Input: part model. Units: mm. Frame: model coordinates. Face numbers are marked on the shaded views. A direction names the side the tool comes from. Give positions to 0.01 mm unless a question says otherwise; leave off trailing zeros. Loops run counter-clockwise (first coordinate to the right, second up) from the corner with the lowest first, then second, coordinate; pieces in that order, holes last.
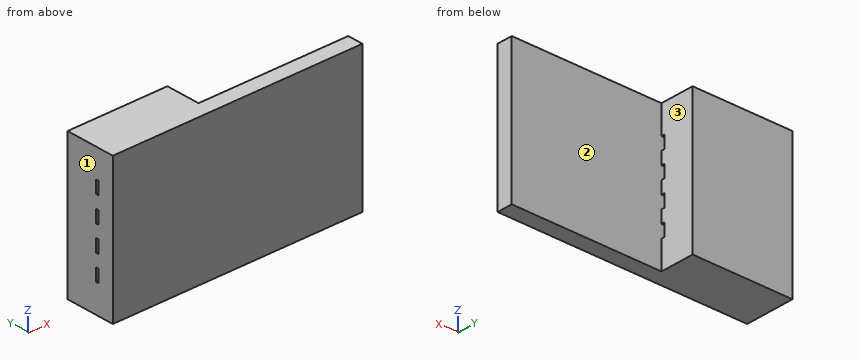
from build123d import *

# Parameters (mm, degrees)
INSULATOR_BODY_SKETCH_W    = 11.5
INSULATOR_BODY_SKETCH_H    = 4
INSULATOR_BODY_DEPTH       = 20
INSULATOR_TONGUE_SKETCH_W  = 12
INSULATOR_TONGUE_SKETCH_H  = 11.5
INSULATOR_TONGUE_DEPTH     = 2.75
CONTACT_SLOT_SKETCH_W      = 1
CONTACT_SLOT_SKETCH_H      = 0.25
CONTACT_SLOT_DEPTH         = 9
CONTACT_SLOT_PATTERN_COUNT = 4
CONTACT_SLOT_PATTERN_PITCH = 2


with BuildPart() as part:
    # Insulator_body_sketch → Insulator_body (new body)
    with BuildSketch(Plane(origin=(0, 0, 0), x_dir=(0, 0, -1), z_dir=(1, 0, 0))):
        Rectangle(INSULATOR_BODY_SKETCH_W, INSULATOR_BODY_SKETCH_H)
    extrude(amount=-INSULATOR_BODY_DEPTH)

    # Insulator_tongue_sketch → Insulator_tongue (cut)
    with BuildSketch(Plane(origin=(0, 2, 0), x_dir=(1, 0, 0), z_dir=(0, 1, 0))):
        with Locations((-6, 0)):
            Rectangle(INSULATOR_TONGUE_SKETCH_W, INSULATOR_TONGUE_SKETCH_H)
    extrude(amount=-INSULATOR_TONGUE_DEPTH, mode=Mode.SUBTRACT)

    # Contact_slot_sketch → Contact_slot (cut, through all)
    with BuildSketch(Plane(origin=(-12, 0, 0), x_dir=(0, 0, -1), z_dir=(1, 0, 0))):
        with Locations((-3, -0.625)):
            Rectangle(CONTACT_SLOT_SKETCH_W, CONTACT_SLOT_SKETCH_H)
    contact_slot = extrude(amount=-CONTACT_SLOT_DEPTH, mode=Mode.SUBTRACT)

    # Contact_slot_pattern: Contact_slot ×4
    with Locations(*[(0, 0, -i * CONTACT_SLOT_PATTERN_PITCH) for i in range(1, CONTACT_SLOT_PATTERN_COUNT)]):
        add(contact_slot, mode=Mode.SUBTRACT)


solid = part.part
(1) Cut plane C-C (y = 0.3). Return the cut outline in (x, z).
Values follow:
outline: (-20, -5.75) - (-12, -5.75) - (-12, 5.75) - (-20, 5.75) - close
(2) Cut plane D-D (x = -3.25). Return the cut outline in (y, z), and give its area (3 significant figures).
Values follow:
outline: (-2, -5.75) - (-0.75, -5.75) - (-0.75, 5.75) - (-2, 5.75) - close
area: 14.4 mm2
(3) Cut plane A-A (z = -1.25). Return the cut outline in (x, y).
Values follow:
outline: (-20, -2) - (0, -2) - (0, -0.75) - (-20, -0.75) - close; (-20, -0.5) - (-12, -0.5) - (-12, 2) - (-20, 2) - close
(4) Ray query, probe 1 along Z at (x, y) = (-14, -0.6); probe 2 along Y at (x, z) = (-17.5, 3); probe 3 along Y at (x, z) = (-2.5, 4.5). Return the intervals inside material, ascending.
Values follow:
probe 1: z = -5.75 to -3.5, -2.5 to -1.5, -0.5 to 0.5, 1.5 to 2.5, 3.5 to 5.75
probe 2: y = -2 to -0.75, -0.5 to 2
probe 3: y = -2 to -0.75
(5) Reachability of the marked faces 1, 2 and 3 from +Z, -Z, +X, -X, +Y, -Y: full face, straight path, thin tool, end or side. Return the list, or none.
Values follow:
face 1: +Z, -Z, -X, +Y, -Y
face 2: +X
face 3: +Z, -Z, +X, +Y
(6) Cut plane B-B (x = -13.75). Return the cut outline in (y, z).
Values follow:
outline: (-2, -5.75) - (2, -5.75) - (2, 5.75) - (-2, 5.75) - close; hole (-0.75, -3.5) - (-0.5, -3.5) - (-0.5, -2.5) - (-0.75, -2.5) - close; hole (-0.75, -1.5) - (-0.5, -1.5) - (-0.5, -0.5) - (-0.75, -0.5) - close; hole (-0.75, 0.5) - (-0.5, 0.5) - (-0.5, 1.5) - (-0.75, 1.5) - close; hole (-0.75, 2.5) - (-0.5, 2.5) - (-0.5, 3.5) - (-0.75, 3.5) - close
(7) Pin query (flat end, axial travel): pin 1 Ø3.5 at (x, z) = (-5, -2.5) entering from +Y; pin 2 Ø2 at (y, z) = (1, 0) entering from +X. Return the tip coordinate at first contact, or that it passes through.
Values follow:
pin 1: stops at y = -0.75
pin 2: stops at x = -12
